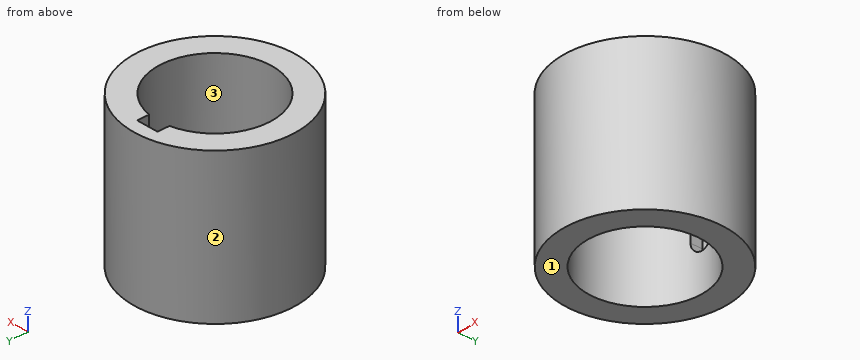
from build123d import *

# Parameters (mm, degrees)
SKETCH1_R           = 18.5
SKETCH1_R_2         = 13
BOSS_EXTRUDE1_DEPTH = 34
SKETCH2_W           = 5
SKETCH2_H           = 5
CUT_EXTRUDE1_DEPTH  = 25.5
FILLET2_R           = 2.5
FILLET3_R           = 2.5


with BuildPart() as part:
    # Sketch1 → Boss-Extrude1 (new body)
    with BuildSketch(Plane.XY):
        Circle(SKETCH1_R)
        Circle(SKETCH1_R_2, mode=Mode.SUBTRACT)
    extrude(amount=BOSS_EXTRUDE1_DEPTH)

    # Sketch2 → Cut-Extrude1 (cut)
    with BuildSketch(Plane.XY.offset(34)):
        with Locations((0, 13)):
            Rectangle(SKETCH2_W, SKETCH2_H)
    extrude(amount=-CUT_EXTRUDE1_DEPTH, mode=Mode.SUBTRACT)

    # Fillet2
    fillet2_edges = [part.edges().sort_by_distance(p)[0] for p in [
        (2.5, 14.128675411, 8.5),
    ]]
    fillet(fillet2_edges, radius=FILLET2_R)

    # Fillet3
    fillet3_edges = [part.edges().sort_by_distance(p)[0] for p in [
        (-2.5, 14.128675411, 8.5),
    ]]
    fillet(fillet3_edges, radius=FILLET3_R - 0.0001)  # a hair under: the kernel refuses the full size


solid = part.part
Input: part model. Units: mm. Frame: model coordinates. Face numbers are marked on the shaded views. Coordinates: 2 decimals unless noted, no trailing zeros. Loops run counter-clockwise (first coordinate to the right, second up) from the corner with the lowest first, then second, coordinate; pieces in that order, holes last.
Q1. Contact query for flat-ended pins moving along their axis: pin 1 (2 mm diameter, centred on x = -15, z = 22.5, fed in from -Y); pin 2 (2.5 mm diameter, centred on x = 0.5, z = 22, fed in from -Y); pin 3 (5 mm diameter, centred on x = -9.5, z = 15, fed in from -Y). Output: stop coordinate, or through.
Q2. Cut plane C-C (y = 6). Output: boundary loops of the cut face in (x, z).
Q3. Cut plane A-A (y = 0). Output: boundary loops of the cut face in (x, z).
Q4. Material intervals for line 1 (X direction, y = -0.5, z = 21.5); line 2 (Y direction, x = 0, z = 26); line 3 (Y direction, x = 0, z = 8), sorted ascending.
Q5. Cut plane D-D (z = 9.5). Output: boundary loops of the cut face in (x, y).
Q6. Draft query along Y for the marked faces 1, 2 and 3. Return one class per face: +Y half, -Y half, draft (parallel to the pull), parting line (faces both ways), or undercut.
Q7. Cut plane B-B (z = 23.5). Output: boundary loops of the cut face in (x, y), then the cut area to 3 significant figures.
Working result:
1. pin 1: stops at y = -12.09
1. pin 2: stops at y = -18.5
1. pin 3: stops at y = -17.12
2. outline: (-17.5, 0) - (-11.53, 0) - (-11.53, 34) - (-17.5, 34) - close; (11.53, 0) - (17.5, 0) - (17.5, 34) - (11.53, 34) - close
3. outline: (-18.5, 0) - (-13, 0) - (-13, 34) - (-18.5, 34) - close; (13, 0) - (18.5, 0) - (18.5, 34) - (13, 34) - close
4. line 1: x = -18.49 to -12.99, 12.99 to 18.49
4. line 2: y = -18.5 to -13, 15.5 to 18.5
4. line 3: y = -18.5 to -13, 13 to 18.5
5. outline: circle Ø37 at (0, 0); hole (-2, 12.85) arc R13 ccw (long way) to (2, 12.85) - (2, 15.5) - (-2, 15.5) - close
6. face 1: draft
6. face 2: parting line
6. face 3: undercut
7. outline: circle Ø37 at (0, 0); hole (-2.5, 12.76) arc R13 ccw (long way) to (2.5, 12.76) - (2.5, 15.5) - (-2.5, 15.5) - close
7. area: 531 mm2
